Autodesk Inventor part; units mm, degrees
ref_plane "Конечная плоскость" through (0, 0, 210) normal (0, 0, 1) x (1, 0, 0)
ref_plane "YZ Plane" through (0, 0, 0) normal (1, 0, 0) x (0, 1, 0)
ref_plane "XZ Plane" through (0, 0, 0) normal (0, 1, 0) x (-1, 0, 0)
sketch "Поручень" plane through (0, 0, 0) normal (0, 0, 1) x (1, 0, 0)
  line L0 (20.3655, -7.6059) -> (20.3655, -0.2092)
  line L1 (20.3655, -0.2092) -> (-19.6345, -0.2092)
  line L2 (-19.6345, -0.2092) -> (-19.6345, -7.6059)
  line L3 (-19.6345, -7.6059) -> (-30.865, -7.6059)
  line L4 (-30.865, -7.6059) -> (-30.865, -5.9622)
  line L5 (-30.865, -5.9622) -> (-32.5087, -5.9622)
  line L6 (-32.5087, -5.9622) -> (-32.5087, 0.6126)
  arc A0 (-30.367, 4.2203) -> (-32.5087, 0.6126) centre (-28.3995, 0.6126) ccw
  arc A1 (-30.367, 4.2203) -> (-30.2973, 18.6123) centre (-34.302, 11.4355) ccw
  arc A2 (-24.2902, 41.7054) -> (-30.2973, 18.6123) centre (-24.2902, 29.3776) ccw
  line L7 (-24.2902, 41.7054) -> (-24.2902, 42.9382)
  arc A3 (25.0211, 42.9382) -> (-24.2902, 42.9382) centre (0.3655, 2.9211) ccw
  line L8 (25.0211, 42.9382) -> (25.0211, 41.7054)
  arc A4 (31.0282, 18.6123) -> (25.0211, 41.7054) centre (25.0211, 29.3776) ccw
  arc A5 (31.0282, 18.6123) -> (31.0979, 4.2203) centre (35.033, 11.4355) ccw
  arc A6 (33.2397, 0.6126) -> (31.0979, 4.2203) centre (29.1304, 0.6126) ccw
  line L9 (33.2397, 0.6126) -> (33.2397, -5.9622)
  line L10 (33.2397, -5.9622) -> (31.596, -5.9622)
  line L11 (31.596, -5.9622) -> (31.596, -7.6059)
  line L12 (31.596, -7.6059) -> (20.3655, -7.6059)
  point P0 (0.3655, -0.2092)
  point P1 (0.3655, -7.6059)
sketch "Эскиз" plane through (0, 0, 0) normal (0, 0, 1) x (1, 0, 0)
  line L0 (20, 0) -> (20, 7.3967)
  line L1 (20, 7.3967) -> (-20, 7.3967)
  line L2 (-20, 7.3967) -> (-20, 0)
  line L3 (-20, 0) -> (-31.2305, 0)
  line L4 (-31.2305, 0) -> (-31.2305, 1.6437)
  line L5 (-31.2305, 1.6437) -> (-32.8742, 1.6437)
  line L6 (-32.8742, 1.6437) -> (-32.8742, 8.2186)
  arc A0 (-30.7325, 11.8262) -> (-32.8742, 8.2186) centre (-28.7649, 8.2186) ccw
  arc A1 (-30.7325, 11.8262) -> (-30.6628, 26.2183) centre (-34.6675, 19.0415) ccw
  arc A2 (-24.6557, 49.3113) -> (-30.6628, 26.2183) centre (-24.6557, 36.9835) ccw
  line L7 (-24.6557, 49.3113) -> (-24.6557, 50.5441)
  arc A3 (24.6557, 50.5441) -> (-24.6557, 50.5441) centre (0, 10.527) ccw
  line L8 (24.6557, 50.5441) -> (24.6557, 49.3113)
  arc A4 (30.6628, 26.2183) -> (24.6557, 49.3113) centre (24.6557, 36.9835) ccw
  arc A5 (30.6628, 26.2183) -> (30.7325, 11.8262) centre (34.6675, 19.0415) ccw
  arc A6 (32.8742, 8.2186) -> (30.7325, 11.8262) centre (28.7649, 8.2186) ccw
  line L9 (32.8742, 8.2186) -> (32.8742, 1.6437)
  line L10 (32.8742, 1.6437) -> (31.2305, 1.6437)
  line L11 (31.2305, 1.6437) -> (31.2305, 0)
  line L12 (31.2305, 0) -> (20, 0)
  point P0 (0, 0)
ref_plane "Начальная плоскость" through (0, 0, 0) normal (0, 0, 1) x (1, 0, 0)
ref_plane "РабПлоскость2" through (0, 0, 210) normal (0, 0, 1) x (1, 0, 0)
extrude "Тело" add sketch "Эскиз" along normal up to surface (210 mm away) from surface at 0
ref_plane "Конечная плоскость" through (0, 0, 210) normal (0, 0, 1) x (1, 0, 0)
equation "\"ШИРИНА\" = 75"
equation "\"ТОЛЩВЫС\" = 58"
equation "\"СЕЧЕНИЕ_СМЕЩ\" = 0"
equation "\"G_OFFSET_END\" = 0"
equation "\"G_OFFSET_START\" = 0"
properties part number "Поручень" material "Древесина (дуб)"
Geometry: final body of the model. Coordinates: model frame, mm. A direction names the side the tool comes from. Round coordinates to 2 decimals unless told otherwise and drop trailing zeros. Loops run counter-clockwise (first coordinate to the right, second up) from the corner with the lowest first, then second, coordinate; pieces in that order, holes last.
Q1. Section B-B on z = 137. Return loops of the section in (x, y).
Q2. Pull-direction query (X, two-part tool) for faces 1 (the flat face through (26, 0, 104)), 2 (the flat face through (20, 4, 104)), 3 (the flat face through (0, 7.397, 104)), 4 (the cylindrical face through (-32.314, 10.29, 103.53)); classes: released by +X, released by -X, zero draft, split by the parting line, or undercut.
Q3. Section D-D on y = 53. Return loops of the section in (x, z).
Q4. Material intervals for L1, parallel to X at y = 3, z = 134.5; L2, parallel to X at y = 36.5, z = 131; L3, parallel to Y at x = -27.5, z = 167.5, sorted ascending.
Q5. Section A-A on y = 4.5. Return loops of the section in (x, z), plus the area to 3 significant figures.
Q6. Access query for faces 5 (the flat face through (-20, 4, 104)), 6 (the flat face through (32.874, 5, 104)), 7 (the flat face through (-32.874, 5, 104)), 8 (the cylindrical face through (32.283, 10.343, 103.53)). Directions: +Z, -Z, +X, -X, +Y, -Y. A direction counts if a zero-diameter tool reaches every point of the face in a straight line with its end or side. Return the directions, or none.
Q7. Section C-C on x = -15.5. Return loops of the section in (y, z), plus the area to 3 significant figures.
Q8. Pin query (flat end, axial travel): P1, Ø1, axis at y = 50, z = 139, coming from the -X side; P2, Ø1.5, axis at x = 26.5, y = 40, coming from the -Z side; P3, Ø5.5, axis at y = 5, z = 146, coming from the -X side; P4, Ø0.5, axis at y = 0.5, z = 139, coming from the -X side. Return the tip coordinate at first contact, or that it passes through.
Evaluation:
1. outline: (-32.87, 1.64) - (-31.23, 1.64) - (-31.23, 0) - (-20, 0) - (-20, 7.4) - (20, 7.4) - (20, 0) - (31.23, 0) - (31.23, 1.64) - (32.87, 1.64) - (32.87, 8.22) arc R4.11 ccw to (30.73, 11.83) arc R8.22 cw to (30.66, 26.22) arc R12.33 ccw to (24.66, 49.31) - (24.66, 50.54) arc R47 ccw to (-24.66, 50.54) - (-24.66, 49.31) arc R12.33 ccw to (-30.66, 26.22) arc R8.22 cw to (-30.73, 11.83) arc R4.11 ccw to (-32.87, 8.22) - close
2. face 1: zero draft
2. face 2: undercut
2. face 3: undercut
2. face 4: released by -X
3. outline: (-20.13, 0) - (20.13, 0) - (20.13, 210) - (-20.13, 210) - close
4. L1: x = -32.87 to -20, 20 to 32.87
4. L2: x = -36.97 to 36.97
4. L3: y = 0 to 15.02, 23.06 to 48.98
5. outline: (-32.87, 0) - (-20, 0) - (-20, 210) - (-32.87, 210) - close; (20, 0) - (32.87, 0) - (32.87, 210) - (20, 210) - close
5. area: 5,410 mm2
6. face 5: +Z, -Z, -Y
6. face 6: +Z, -Z, +X, -Y
6. face 7: +Z, -Z, -X, -Y
6. face 8: +Z, -Z, +X
7. outline: (7.4, 0) - (54.9, 0) - (54.9, 210) - (7.4, 210) - close
7. area: 9,980 mm2
8. P1: stops at x = -24.66
8. P2: stops at z = 0
8. P3: stops at x = -32.87
8. P4: stops at x = -31.23
